from build123d import *

# Parameters (mm, degrees)
SKETCH1_R           = 5
SKETCH1_R_2         = 3
BOSS_EXTRUDE1_DEPTH = 4
SKETCH2_R           = 0.5
CUT_EXTRUDE1_DEPTH  = 5
BOSS_EXTRUDE2_DEPTH = 4


with BuildPart() as part:
    # Sketch1 → Boss-Extrude1 (new body)
    with BuildSketch(Plane(origin=(0, 0, 0), x_dir=(1, 0, 0), z_dir=(0, 1, 0))):
        with Locations((-1, 0)):
            Circle(SKETCH1_R)
        Circle(SKETCH1_R_2, mode=Mode.SUBTRACT)
    extrude(amount=BOSS_EXTRUDE1_DEPTH)

    # Sketch2 → Cut-Extrude1 (cut, through all)
    with BuildSketch(Plane(origin=(0, 4, 0), x_dir=(1, 0, 0), z_dir=(0, 1, 0))):
        with Locations((0, 3.75)):
            Circle(SKETCH2_R)
        with Locations((0, -3.75)):
            Circle(SKETCH2_R)
    extrude(amount=-CUT_EXTRUDE1_DEPTH, mode=Mode.SUBTRACT)

    # Sketch3 → Boss-Extrude2 (add)
    with BuildSketch(Plane.XZ):
        with BuildLine():
            ThreePointArc((3, 0), (2.738612788, 1.224744871), (2, 2.236067977))
            Line((2, 2.236067977), (2, -2.236067977))
            ThreePointArc((2, -2.236067977), (2.738612788, -1.224744871), (3, 0))
        make_face()
    extrude(amount=-BOSS_EXTRUDE2_DEPTH)


solid = part.part
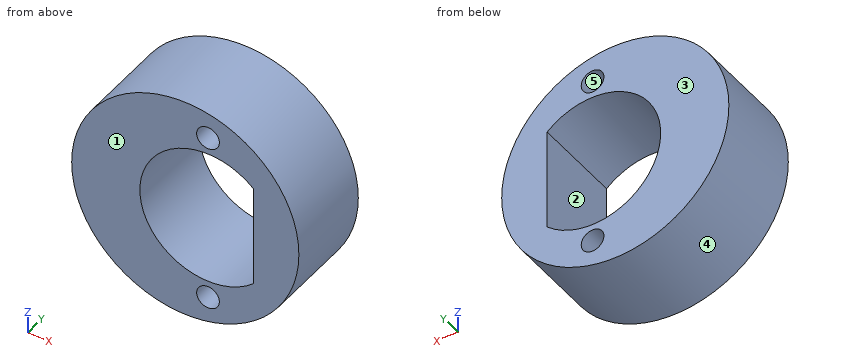
Model file for the job. Use its own axes, mm. Face numbers are marked on the shaded views. A direction names the side the tool comes from. Give positions to 0.01 mm unless a question says otherwise; leave off trailing zeros. Loops run counter-clockwise (first coordinate to the right, second up) from the corner with the lowest first, then second, coordinate; pieces in that order, holes last.
Item 1: Slice it at C-C (z = -0.25). Write the cut outline in (x, y).
Check values:
outline: (-5.99, 0) - (-2.99, 0) - (-2.99, 4) - (-5.99, 4) - close; (2, 0) - (3.99, 0) - (3.99, 4) - (2, 4) - close
Item 2: Mould opens along Z. For the marked faces 3, 4 and 5 say: +Z half, -Z half, draft (parallel to the pull), parting line (faces both ways), or undercut.
Check values:
face 3: draft
face 4: parting line
face 5: undercut
Item 3: Which spindle directions (+Z, -Z, +X, -X, +Y, -Y) get a long thin tool onto all of the face, cutting with end or side? Do the marked faces 1 and 2. Say none if no direction does.
Check values:
face 1: +Z, -Z, +X, -X, -Y
face 2: +Y, -Y
Item 4: Slice it at D-D (y = 0.3). Write the cut outline in (x, z).
Check values:
outline: circle Ø10 at (-1, 0); hole circle Ø1 at (0, -3.75); hole circle Ø1 at (0, 3.75); hole (2, -2.24) - (2, 2.24) arc R3 ccw (long way) to start
Item 5: Slice it at A-A (x = -1.75). Write the cut outline in (y, z), plus the area to 3 significant figures.
Check values:
outline: (0, -4.94) - (4, -4.94) - (4, -2.44) - (0, -2.44) - close; (0, 2.44) - (4, 2.44) - (4, 4.94) - (0, 4.94) - close
area: 20.1 mm2
Item 6: Drill centre lines: line 1 along Z through (x, y) = (0, 2.4); line 2 along X through (y, z) = (1.5, 1); line 3 along X through (y, z) = (2.45, 0.5). Where is each one in solid material? Low to high.
Check values:
line 1: z = -4.9 to -4.25, -3.25 to -3, 3 to 3.25, 4.25 to 4.9
line 2: x = -5.9 to -2.83, 2 to 3.9
line 3: x = -5.97 to -2.96, 2 to 3.97
Item 7: Slice it at B-B (x = 0). Write the cut outline in (y, z), plus the area to 3 significant figures.
Check values:
outline: (0, -4.9) - (4, -4.9) - (4, -4.25) - (0, -4.25) - close; (0, -3.25) - (4, -3.25) - (4, -3) - (0, -3) - close; (0, 3) - (4, 3) - (4, 3.25) - (0, 3.25) - close; (0, 4.25) - (4, 4.25) - (4, 4.9) - (0, 4.9) - close
area: 7.19 mm2
Item 8: Drop a flat-ended pin along its axis: P1, Ø1, axis at x = -3, y = 1.5, coming from the -Z side. Give the stop position or say it passes through.
Check values:
P1: stops at z = -4.77
